from build123d import *

# Parameters (mm, degrees)
SCHIZZO1_W                   = 35
SCHIZZO1_H                   = 19
SCHIZZO1_R                   = 4
ESTRUSIONE_ESTRUSIONE1_DEPTH = 6.35


with BuildPart() as part:
    # Schizzo1 → Estrusione-Estrusione1 (new body)
    with BuildSketch(Plane(origin=(0, 0, 0), x_dir=(1, 0, 0), z_dir=(0, 1, 0))):
        Rectangle(SCHIZZO1_W, SCHIZZO1_H)
        with Locations(Location((-8, 0.5, 0), (0, 0, 270))):
            Circle(SCHIZZO1_R, mode=Mode.SUBTRACT)
    extrude(amount=ESTRUSIONE_ESTRUSIONE1_DEPTH)


solid = part.part
The model under review builds one solid part; all positions refer to its coordinate system, in mm. Give positions to 0.01 mm unless a question says otherwise; leave off trailing zeros. Loops run counter-clockwise (first coordinate to the right, second up) from the corner with the lowest first, then second, coordinate; pieces in that order, holes last. Notation, with made-up numbers: (23.5, -16) -> (73.5, -16) arc R19 ccw to (73.5, 4) -> close; hole circle Ø10 at (34, -33). An arc over 180 degrees is marked (long way). Answer as a JSON object with one key per item and string values. Group by question number.
Q1. Draft analysis for pull direction Z (two halves, no side actions). For faces 1 (the flat face through (0, 3, 9.5)), 2 (the flat face through (0, 6.35, 0)), 3 (the cylindrical face through (-11.549, 3.131, 1.346)), 4 (the flat face through (0, 3, -9.5)), state which applies: pulls with the +Z half, pulls with the -Z half, needs draft (parallel to the pull), parting line crosses it, or undercut.
Q2. Insertion check: pin 1 (4 mm diameter, centred on x = -9, z = 0.5, fed in from +Y). The pin has a flat end and moves straight along its axis. Give the tip position at first contact, or say it passes through.
Q3. Take a section at B-B (z = -0.5). Write out the cut boundary in (x, y).
Q4. Wall thickness on line 1 along X through (y, z) = (1.75, -0.5); line 2 along X through (y, z) = (5, -3.5); line 3 along Z through (x, y) = (-6, 5.75): over which ranges is each line inside the solid? List them lowest first.
Q5. Take a section at C-C (y = 4.5). Write out the cut boundary in (x, z).
Q6. Take a section at A-A (x = -8). Write out the cut boundary in (y, z), plus the area to 4 significant figures.
Answer below:
{
 "1": {"face 1": "pulls with the +Z half", "face 2": "needs draft", "face 3": "undercut", "face 4": "pulls with the -Z half"},
 "2": {"pin 1": "passes through"},
 "3": {"outline": "(-17.5, 0) -> (-12, 0) -> (-12, 6.35) -> (-17.5, 6.35) -> close; (-4, 0) -> (17.5, 0) -> (17.5, 6.35) -> (-4, 6.35) -> close"},
 "4": {"line 1": "x = -17.5 to -12, -4 to 17.5", "line 2": "x = -17.5 to -10.65, -5.35 to 17.5", "line 3": "z = -9.5 to -3.96, 2.96 to 9.5"},
 "5": {"outline": "(-17.5, -9.5) -> (17.5, -9.5) -> (17.5, 9.5) -> (-17.5, 9.5) -> close; hole circle Ø8 at (-8, -0.5)"},
 "6": {"outline": "(0, -9.5) -> (6.35, -9.5) -> (6.35, -4.5) -> (0, -4.5) -> close; (0, 3.5) -> (6.35, 3.5) -> (6.35, 9.5) -> (0, 9.5) -> close", "area": "69.85 mm2"}
}
